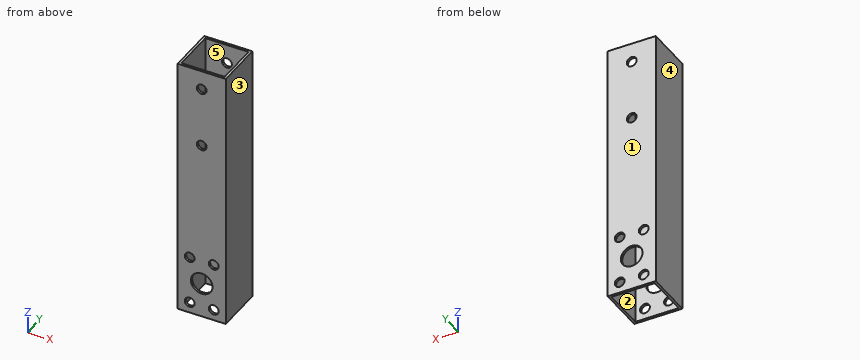
```python
from build123d import *

# Parameters (mm, degrees)
SKETCH_1_2_W         = 20
SKETCH_1_2_H         = 20
SKETCH_1_2_W_2       = 18
SKETCH_1_2_H_2       = 18
EXTRUDE_2_DEPTH      = 54.5
SKETCH_2_R           = 2.05
CUT_EXTRUDE_1_DEPTH  = 102
SKETCH_11_R          = 2.05
CUT_EXTRUDE_8_DEPTH  = 50
SKETCH_17_R          = 4.5
CUT_EXTRUDE_14_DEPTH = 40


with BuildPart() as part:
    # Sketch 1_2 → Extrude 2 (new, symmetric)
    with BuildSketch(Plane.XY):
        Rectangle(SKETCH_1_2_W, SKETCH_1_2_H)
        Rectangle(SKETCH_1_2_W_2, SKETCH_1_2_H_2, mode=Mode.SUBTRACT)
    extrude(amount=EXTRUDE_2_DEPTH, both=True)

    # Sketch 2 → Cut-Extrude 1 (cut)
    with BuildSketch(Plane(origin=(0, 10, 0), x_dir=(1, 0, 0), z_dir=(0, 1, 0))):
        with Locations(Location((0, -46.5, 0), (0, 0, 270))):
            Circle(SKETCH_2_R)
        with Locations(Location((0, -21.5, 0), (0, 0, 270))):
            Circle(SKETCH_2_R)
    extrude(amount=-CUT_EXTRUDE_1_DEPTH, mode=Mode.SUBTRACT)

    # Sketch 11 → Cut-Extrude 8 (cut)
    with BuildSketch(Plane(origin=(0, 10, 0), x_dir=(1, 0, 0), z_dir=(0, 1, 0))):
        with Locations(Location((5, 29.933387088, 0), (0, 0, 270))):
            Circle(SKETCH_11_R)
        with Locations(Location((-5, 29.933387088, 0), (0, 0, 270))):
            Circle(SKETCH_11_R)
        with Locations(Location((5, 49.933387088, 0), (0, 0, 270))):
            Circle(SKETCH_11_R)
        with Locations(Location((-5, 49.933387088, 0), (0, 0, 270))):
            Circle(SKETCH_11_R)
    extrude(amount=-CUT_EXTRUDE_8_DEPTH, mode=Mode.SUBTRACT)

    # Sketch 17 → Cut-Extrude 14 (cut)
    with BuildSketch(Plane(origin=(0, 10, 0), x_dir=(1, 0, 0), z_dir=(0, 1, 0))):
        with Locations(Location((0, 39.933387088, 0), (0, 0, 270))):
            Circle(SKETCH_17_R)
    extrude(amount=-CUT_EXTRUDE_14_DEPTH, mode=Mode.SUBTRACT)


solid = part.part
```
The model under review builds one solid part; all positions refer to its coordinate system, in mm. Face numbers are marked on the shaded views. A direction names the side the tool comes from. Give positions to 0.01 mm unless a question says otherwise; leave off trailing zeros. Write each loop counter-clockwise with the first axis right and the second up, starting at its lowest first coordinate (ties: lowest second). Pieces come first, ordered by that corner, then holes. Notation, with made-up numbers: M 17,-21 L 50,-21 A18 cw 50,11 Z; hole C 37.25,11 d5. An arc over 180 degrees is marked long. Write each question's results on one line, items separated by ' | '. Start each with the question number.
1. Insertion check: pin 1 Ø3.5 at (x, z) = (-5, -29.93) entering from +Y. The pin has a flat end and moves straight along its axis. Give the tip position at first contact, or say it passes through.
2. We need section D-D (z = -14.5). Write out the cut boundary in (x, y), and give its area (3 significant figures).
3. Mouldability with a two-part tool opening along X and no side actions: class the marked faces 1, 2 and 3 as released by +X, released by -X, zero draft, split by the parting line, or undercut.
4. For probe 1 along X at (y, z) = (3.75, 4.5), list the stretches that pass through material, from the lowest coordinate up. Write a range as [from, to].
5. We need section C-C (y = -8). Write out the cut boundary in (x, z), and give its area (3 significant figures).
6. For the marked faces 4 and 5, list the 3-axis set-ups (+Z, -Z, +X, -X, +Y, -Y) from which the entire face can be reached by the end or side of a thin tool; tool diameter is ignored.
7. We need section A-A (x = 0). Count the separate pieces of the cut face and the enclosed holes in it, and give its area (3 significant figures).
8. We need section B-B (z = 21.5). Write out the cut boundary in (x, y), and give its area (3 significant figures).
Results found:
1) pin 1: passes through
2) outline: M -10,-10 L 10,-10 L 10,10 L -10,10 Z; hole M -9,-9 L 9,-9 L 9,9 L -9,9 Z | area: 76.0 mm^2
3) face 1: zero draft | face 2: undercut | face 3: released by +X
4) probe 1: x = [-10, -9], [9, 10]
5) outline: M -10,-54.5 L -9,-54.5 L -9,54.5 L -10,54.5 Z; M 9,-54.5 L 10,-54.5 L 10,54.5 L 9,54.5 Z | area: 218 mm^2
6) face 4: +Z, -Z, -X, +Y, -Y | face 5: +Z, -Z
7) separate pieces: 8 | enclosed holes: 0 | area: 184 mm^2
8) outline: M -10,-10 L -2.05,-10 L -2.05,-9 L -9,-9 L -9,9 L -2.05,9 L -2.05,10 L -10,10 Z; M 2.05,-10 L 10,-10 L 10,10 L 2.05,10 L 2.05,9 L 9,9 L 9,-9 L 2.05,-9 Z | area: 67.8 mm^2
